Answer from the drawing. Dimensions are ordinates in mm from the lowest x, y and z of the part. A direction names the side the tool comes from. Give positions to 0.01 mm unless a question says otherwise; leave off trailing zeros. Write each loop counter-clockwise with the first axis right and the second up, starting at its lowest first coordinate (ties: lowest second). Pieces come first, ordered by that corner, then holes.
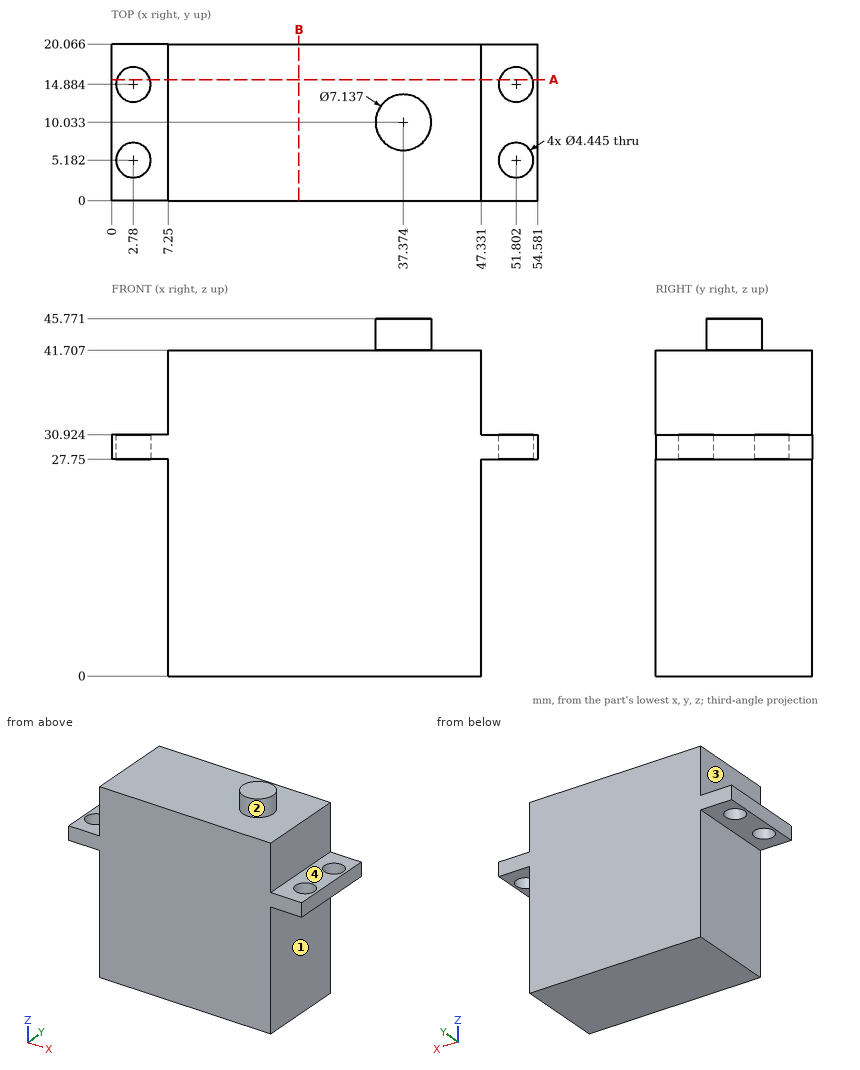
Item 1: Section A-A (y = 15.5) is taken. Give the number of separate pieces and of enclosed holes in the cut face, and give its area (3 significant figures).
Result set:
separate pieces: 3
enclosed holes: 0
area: 1,690 mm2
Item 2: Find the intervals of material crossed by line 1 along Z through (x, y) = (15, 3.75); line 2 along X through (y, z) = (12.5, 15); line 3 along X through (y, z) = (7, 43) (1 decimal), in increasing order.
Result set:
line 1: z = 0 to 41.71
line 2: x = 7.25 to 47.33
line 3: x = 35.5 to 39.3
Item 3: Section B-B (x = 24) is taken. Write down the section's boundary in (y, z) (1 decimal).
Result set:
outline: (0, 0) - (20.1, 0) - (20.1, 41.7) - (0, 41.7) - close
Item 4: Which of the six approach directions +Z, -Z, +X, -X, +Y, -Y give full straight-line access (tool end or side, diameter ignored) to the marked faces 1, 2, 3 and 4?
Result set:
face 1: -Z, +X, +Y, -Y
face 2: +Z
face 3: +Z, -X, +Y, -Y
face 4: +Z, +X, +Y, -Y
Item 5: Each of these flat-tipped pins is pushed along its axis until it touches: pin 1 Ø8 at (x, y) = (2, 12.5) entering from -Z; pin 2 Ø4 at (x, y) = (2.78, 14.88) entering from -Z; pin 3 Ø8 at (x, y) = (25.5, 17) entering from +Z; pin 4 Ø10 at (y, z) = (12, 10) entering from -X. Where does it stop, or does it pass through?
Result set:
pin 1: stops at z = 27.75
pin 2: passes through
pin 3: stops at z = 41.71
pin 4: stops at x = 7.25
